Could you check a few things on this drawing? It's one solid part, dimensions in mm from its lowest x, y, z. Coordinates: 2 decimals unless noted, no trailing zeros. Write each loop counter-clockwise with the first axis right and the second up, starting at its lowest first coordinate (ties: lowest second). Pieces come first, ordered by that corner, then holes. Notation, with made-up numbers: (-26, 41.5) - (33, 41.5) arc R25 cw to (33, 68.5) - close; hole circle Ø10 at (16.5, 33). An arc over 180 degrees is marked (long way). Answer as a JSON object with one key per item and string values. Group by question number.
1) If we section it at B-B (z = 1): Write out the boundary of the cut face in (x, y) (1 decimal), plus the area to 3 significant figures.
2) We'd pull the mould along Z, two halves only. Please class the marked faces 1, 2 and 3: released by +Z, released by -Z, zero draft, split by the parting line, or undercut.
3) If we section it at A-A (z = 3.5): Write out the boundary of the cut face in (x, y), plus the area to 3 significant figures.
4) Please list where these lines run through material, in increasing order: line 1 along Y through (x, z) = (6, 4) (1 decimal); line 2 along Y through (x, z) = (9, 6.5) (1 decimal); line 3 along X through (y, z) = (9.25, 2.5).
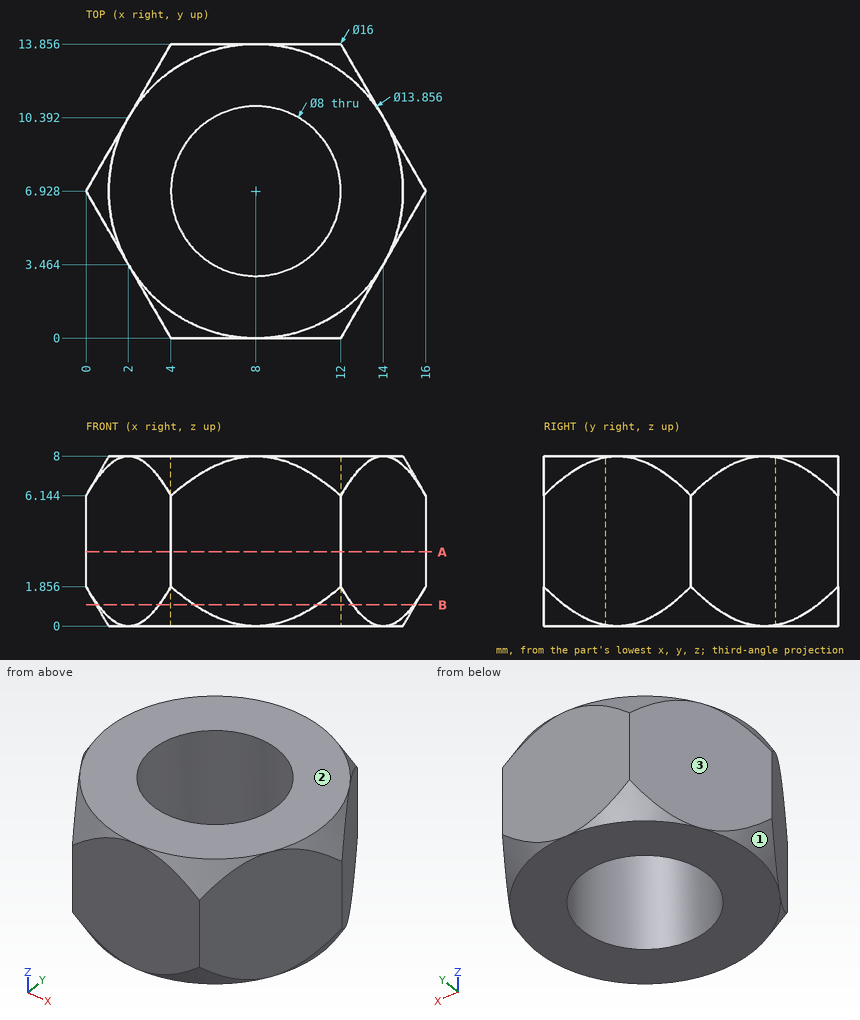
Here are the results:
{
 "1": {"outline": "(0.6, 6) - (3.4, 1) arc R7.5 ccw to (5.1, 0) - (10.9, 0) arc R7.5 ccw to (12.6, 1) - (15.4, 6) arc R7.5 ccw to (15.4, 7.9) - (12.6, 12.9) arc R7.5 ccw to (10.9, 13.9) - (5.1, 13.9) arc R7.5 ccw to (3.4, 12.9) - (0.6, 7.9) arc R7.5 ccw to start; hole circle Ø8 at (8, 6.9)", "area": "113 mm²"},
 "2": {"face 1": "released by -Z", "face 2": "released by +Z", "face 3": "zero draft"},
 "3": {"outline": "(0, 6.93) - (4, 0) - (12, 0) - (16, 6.93) - (12, 13.86) - (4, 13.86) - close; hole circle Ø8 at (8, 6.93)", "area": "116 mm²"},
 "4": {"line 1": "y = 0 to 3.5, 10.4 to 13.9", "line 2": "y = 0 to 3.1, 10.8 to 13.9", "line 3": "x = 1.34 to 4.74, 11.26 to 14.66"}
}
